Verification items for the finished model (mm, model axes). A direction names the side the tool comes from. Coordinates: 2 decimals unless noted, no trailing zeros. Loops run counter-clockwise (first coordinate to the right, second up) from the corner with the lowest first, then second, coordinate; pieces in that order, holes last. Notation, with made-up numbers: (9, -19) - (17, -19) arc R19 ccw to (17, 10) - close; hole circle Ø7 at (13, 39.5). An arc over 180 degrees is marked (long way). One line per item, written item: value. Start each with the question number.
(1) Section check D-D (z = 23.5). Record the boundary of the cut face in (x, y).
(2) Set-up check for faces 4 (the face through (26.61, -0.99, 34.7)), 5 (the face through (28.771, -0.986, -14.827)): record each of +Z, -Z, +X, -X, +Y, -Y from which the full face is reachable in a straight line by a thin tool's end or side.
(3) Draft check along X on faces 1 (the face through (-1, -2, 6)), 2 (the face through (-44.26, -0.99, 3.16)), 3 (the face through (-26.254, -0.986, 34.731)). Enter one of: +X half, -X half, draft (parallel to the pull), parting line (faces both ways), or undercut.
(4) Section check C-C (x = 36). Record the boundary of the cut face in (y, z).
(5) Gauge pin test, flat ends, axial feed: P1, Ø0.6, axis at y = -1, z = 6, coming from the -X side; P2, Ø1, axis at y = -1, z = -8.5, coming from the +X side; P3, Ø1, axis at x = -60, y = -1.5, coming from the -Z side. Record the tip position at first contact, or that the pin passes through.
(6) Thickness scan on probe 1 along X at (y, z) = (-1.8, 13.5); probe 2 along X at (y, z) = (-1.4, 26); probe 3 along X at (y, z) = (-0.15, -9.5). Record the ranges inside material, lowest first. Write a range as [from, to].
(7) Section check A-A (z = 9). Record the boundary of the cut face in (x, y).
(8) Section check B-B (z = -3). Record the boundary of the cut face in (x, y), plus the area to 3 significant figures.
```python
from build123d import *

# Parameters (mm, degrees)
F0_W     = 2
F0_H     = 11
F1_DEPTH = 2


with BuildPart() as f1:
    # F0 (on Front) → F1 (new body)
    with BuildSketch(Plane.XZ):
        with BuildLine():
            Line((0.144111, 35.317095), (-19.580889, 35.317095))
            Line((-19.580889, 35.317095), (-21.580889, 35.317095))
            Line((-21.580889, 35.317095), (-23.668159, 35.317095))
            ThreePointArc((-23.668159, 35.317095), (-26.28845, 34.714694), (-28.382586, 33.028452))
            Line((-28.382586, 33.028452), (-62.295316, -10.04988))
            ThreePointArc((-62.295316, -10.04988), (-63.250393, -11.797385), (-63.580889, -13.761238))
            Line((-63.580889, -13.761238), (-63.580889, -21.682905))
            Line((-63.580889, -21.682905), (-53.580889, -21.682905))
            Line((-53.580889, -21.682905), (-53.580889, -23.682905))
            Line((-53.580889, -23.682905), (-39.080889, -23.682905))
            Line((-39.080889, -23.682905), (-39.080889, -21.682905))
            Line((-39.080889, -21.682905), (-21.580889, -21.682905))
            Line((-21.580889, -21.682905), (-7.330889, -21.682905))
            Line((-7.330889, -21.682905), (-7.330889, -21.849002))
            Line((-7.330889, -21.849002), (-7.330889, -23.682905))
            Line((-7.330889, -23.682905), (0.144111, -23.682905))
            Line((0.144111, -23.682905), (0.144111, 20.317095))
            ThreePointArc((0.144111, 20.317095), (-4.855889, 25.317095), (0.144111, 30.317095))
            Line((0.144111, 30.317095), (0.144111, 35.317095))
        make_face()
        with Locations((-20.580889, -10.349002)):
            Rectangle(F0_W, F0_H, mode=Mode.SUBTRACT)
        with BuildLine():
            Line((-30.580889, -15.682905), (-52.913921, -15.682905))
            ThreePointArc((-52.913921, -15.682905), (-55.612721, -13.993051), (-55.271135, -10.827226))
            Line((-55.271135, -10.827226), (-32.938102, 17.541761))
            ThreePointArc((-32.938102, 17.541761), (-29.598962, 18.520834), (-27.580889, 15.686082))
            Line((-27.580889, 15.686082), (-27.580889, -12.682905))
            ThreePointArc((-27.580889, -12.682905), (-28.459568, -14.804226), (-30.580889, -15.682905))
        make_face(mode=Mode.SUBTRACT)
        with Locations((-20.580889, 6.817095)):
            Rectangle(F0_W, F0_H, mode=Mode.SUBTRACT)
        with Locations((-20.580889, 23.817095)):
            Rectangle(F0_W, F0_H, mode=Mode.SUBTRACT)
        with BuildLine():
            Line((19.869111, 35.317095), (0.144111, 35.317095))
            Line((0.144111, 35.317095), (0.144111, 30.317095))
            ThreePointArc((0.144111, 30.317095), (3.679645, 28.852629), (5.144111, 25.317095))
            ThreePointArc((5.144111, 25.317095), (3.679645, 21.781561), (0.144111, 20.317095))
            Line((0.144111, 20.317095), (0.144111, -23.682905))
            Line((0.144111, -23.682905), (7.619111, -23.682905))
            Line((7.619111, -23.682905), (7.619111, -21.849002))
            Line((7.619111, -21.849002), (7.619111, -21.682905))
            Line((7.619111, -21.682905), (21.869111, -21.682905))
            Line((21.869111, -21.682905), (39.369111, -21.682905))
            Line((39.369111, -21.682905), (39.369111, -23.682905))
            Line((39.369111, -23.682905), (53.869111, -23.682905))
            Line((53.869111, -23.682905), (53.869111, -21.682905))
            Line((53.869111, -21.682905), (63.869111, -21.682905))
            Line((63.869111, -21.682905), (63.869111, -13.761238))
            ThreePointArc((63.869111, -13.761238), (63.538616, -11.797385), (62.583538, -10.04988))
            Line((62.583538, -10.04988), (28.670808, 33.028452))
            ThreePointArc((28.670808, 33.028452), (26.576673, 34.714694), (23.956381, 35.317095))
            Line((23.956381, 35.317095), (21.869111, 35.317095))
            Line((21.869111, 35.317095), (19.869111, 35.317095))
        make_face()
        with Locations((20.869111, -10.349002)):
            Rectangle(F0_W, F0_H, mode=Mode.SUBTRACT)
        with BuildLine():
            Line((53.202144, -15.682905), (30.869111, -15.682905))
            ThreePointArc((30.869111, -15.682905), (28.747791, -14.804226), (27.869111, -12.682905))
            Line((27.869111, -12.682905), (27.869111, 15.686082))
            ThreePointArc((27.869111, 15.686082), (29.887185, 18.520834), (33.226325, 17.541761))
            Line((33.226325, 17.541761), (55.559357, -10.827226))
            ThreePointArc((55.559357, -10.827226), (55.900943, -13.993051), (53.202144, -15.682905))
        make_face(mode=Mode.SUBTRACT)
        with Locations((20.869111, 6.817095)):
            Rectangle(F0_W, F0_H, mode=Mode.SUBTRACT)
        with Locations((20.869111, 23.817095)):
            Rectangle(F0_W, F0_H, mode=Mode.SUBTRACT)
    extrude(amount=F1_DEPTH)


solid = f1.part
```
Responses:
1. outline: (-35.88, -2) - (-21.58, -2) - (-21.58, 0) - (-35.88, 0) - close; (-19.58, -2) - (-4.51, -2) - (-4.51, 0) - (-19.58, 0) - close; (4.8, -2) - (19.87, -2) - (19.87, 0) - (4.8, 0) - close; (21.87, -2) - (36.17, -2) - (36.17, 0) - (21.87, 0) - close
2. face 4: +Z, +X, +Y, -Y
2. face 5: +Y, -Y
3. face 1: draft
3. face 2: undercut
3. face 3: -X half
4. outline: (-2, -21.68) - (0, -21.68) - (0, -15.68) - (-2, -15.68) - close; (-2, 14.02) - (0, 14.02) - (0, 23.72) - (-2, 23.72) - close
5. P1: stops at x = -49.9
5. P2: stops at x = 61.76
5. P3: stops at z = -21.68
6. probe 1: x = [-43.76, -36.12], [-27.58, 27.87], [36.41, 44.04]
6. probe 2: x = [-33.92, -21.58], [-19.58, -4.81], [5.1, 19.87], [21.87, 34.2]
6. probe 3: x = [-61.86, -54.23], [-27.58, -21.58], [-19.58, 19.87], [21.87, 27.87], [54.51, 62.15]
7. outline: (-47.3, -2) - (-39.66, -2) - (-39.66, 0) - (-47.3, 0) - close; (-27.58, -2) - (-21.58, -2) - (-21.58, 0) - (-27.58, 0) - close; (-19.58, -2) - (19.87, -2) - (19.87, 0) - (-19.58, 0) - close; (21.87, -2) - (27.87, -2) - (27.87, 0) - (21.87, 0) - close; (39.95, -2) - (47.59, -2) - (47.59, 0) - (39.95, 0) - close
8. outline: (-56.75, -2) - (-49.11, -2) - (-49.11, 0) - (-56.75, 0) - close; (-27.58, -2) - (27.87, -2) - (27.87, 0) - (-27.58, 0) - close; (49.4, -2) - (57.03, -2) - (57.03, 0) - (49.4, 0) - close
8. area: 141 mm²
